The model under review builds one solid part; all positions refer to its coordinate system, in mm. Face numbers are marked on the shaded views. Round coordinates to 2 decimals unless told otherwise and drop trailing zeros. Write each loop counter-clockwise with the first axis right and the second up, starting at its lowest first coordinate (ties: lowest second). Pieces come first, ordered by that corner, then holes.
Item 1: To check wall thickness, follow L1, parallel to Z at x = 17, y = -10; L2, parallel to Z at x = 17.25, y = -72.5; L3, parallel to Y at x = 20.25, z = -44. State the ranges of each line that lie inside material, in increasing order.
Item 2: Draft analysis for pull direction Y (two halves, no side actions). For the marked faces 1, 2, 3 and 4, state which applies: +Y half, -Y half, draft (parallel to the pull), parting line (faces both ways), or undercut.
Item 3: Add section C-C (y = -47.5). Give the boundary of the cut face in (x, z).
Item 4: Add section A-A (x = 12.5). State how many separate pieces and enclosed holes the cut face has, plus the area to 3 significant figures.
Item 5: Add section B-B (y = -10). Give the boundary of the cut face in (x, z), plus the area to 3 significant figures.
Item 6: Clearance check with flat-ended pins moving along their axes: pin 1 Ø5 at (x, y) = (6, -58.5) entering from +Z; pin 2 Ø2 at (y, z) = (-10.5, -35.5) entering from -X; pin 3 Ø13 at (y, z) = (-97.5, -15.95) entering from +X; pin 4 Ø5.5 at (y, z) = (-10, -11) entering from +X. State where each tip first meets the part, or that it passes through.
Item 7: Add section D-D (z = -46). Give the boundary of the cut face in (x, y), plus the area to 4 significant figures.
Autodesk Inventor part; units mm, degrees
ref_plane "YZ Plane" through (0, 0, 0) normal (1, 0, 0) x (0, 1, 0)
ref_plane "XZ Plane" through (0, 0, 0) normal (0, 1, 0) x (-1, 0, 0)
ref_plane "XY Plane" through (0, 0, 0) normal (0, 0, 1) x (1, 0, 0)
sketch "Sketch1" plane through (0, 0, 0) normal (1, 0, 0) x (0, 1, 0)
  line L0 (0, 0) -> (-145, 0)
  line L1 (-145, 0) -> (-145, -70)
  line L2 (-145, -70) -> (0, -70)
  line L3 (0, -70) -> (0, 0)
  dimension "d0" = 145
  dimension "d1" = 70
extrude "Extrusion1" add sketch "Sketch1" along normal blind 20
sketch "Sketch5" plane through (20, 0, 0) normal (1, 0, 0) x (0, 0, -1)
  line L0 (49.9481, -33) -> (-5.5519, -33)
  arc A0 (-6.6519, -32.6703) -> (-5.5519, -33) centre (-5.5519, -31) ccw
  line L1 (-6.6519, -32.6703) -> (-6.6519, -47)
  arc A1 (-9.5519, -49.9) -> (-6.6519, -47) centre (-9.5519, -47) ccw
  line L2 (-9.5519, -49.9) -> (-23.8816, -49.9)
  arc A2 (-23.5519, -51) -> (-23.8816, -49.9) centre (-25.5519, -51) ccw
  line L3 (-23.5519, -51) -> (-23.5519, -106.5)
  arc A3 (-23.5519, -106.5) -> (-18.0519, -112) centre (-18.0519, -106.5) ccw
  line L4 (-18.0519, -112) -> (49.9481, -112)
  arc A4 (49.9481, -112) -> (55.4481, -106.5) centre (49.9481, -106.5) ccw
  line L5 (55.4481, -106.5) -> (55.4481, -38.5)
  arc A5 (55.4481, -38.5) -> (49.9481, -33) centre (49.9481, -38.5) ccw
  circle A6 centre (15.9481, -97.5) radius 1.65
  circle A7 centre (15.9481, -47.5) radius 1.65
  circle A8 centre (50.6979, -96.4808) radius 0.6924
  circle A9 centre (-9.0519, -72.5) radius 5.5
  circle A10 centre (40.9481, -72.5) radius 5.5
  circle A11 centre (15.9481, -72.5) radius 2.5
  circle A12 centre (-9.0519, -97.5) radius 4
  circle A13 centre (40.9481, -47.5) radius 4
  circle A14 centre (28.9481, -89.75) radius 1.5
  circle A15 centre (47.9481, -43.6) radius 1.5
  circle A16 centre (-12.9519, -104.5) radius 1.5
  circle A17 centre (33.1981, -85.5) radius 1.5
  circle A18 centre (-1.8019, -49.6) radius 1.5
  circle A19 centre (-6.9519, -54.75) radius 1.5
  line L6 (43.2888, -99.6225) -> (54.231, -96.5)
  line L7 (54.231, -96.5) -> (50.8902, -107.3775)
  line L8 (50.8902, -107.3775) -> (39.9481, -110.5)
  line L9 (39.9481, -110.5) -> (43.2888, -99.6225)
  line L10 (49.9481, -32.5) -> (-5.5519, -32.5)
  arc A20 (55.9481, -38.5) -> (49.9481, -32.5) centre (49.9481, -38.5) ccw
  line L11 (55.9481, -106.5) -> (55.9481, -38.5)
  arc A21 (49.9481, -112.5) -> (55.9481, -106.5) centre (49.9481, -106.5) ccw
  line L12 (-18.0519, -112.5) -> (49.9481, -112.5)
sketch "Sketch10" plane through (20, 0, 0) normal (1, 0, 0) x (0, 0, -1)
  line L0 (0, 0) -> (0, -145) construction
  line L1 (0, -145) -> (70, -145) construction
  line L2 (70, -145) -> (70, 0) construction
  line L3 (70, 0) -> (0, 0) construction
  line L4 (49.9481, -32.5) -> (-5.5519, -32.5) construction
  line L5 (55.9481, -106.5) -> (55.9481, -38.5) construction
  line L6 (-18.0519, -112.5) -> (49.9481, -112.5) construction
  line L7 (0, 0) -> (0, -145) construction
  line L8 (0, -112.5) -> (0, -145)
  line L9 (0, -145) -> (70, -145)
  line L10 (0, -145) -> (70, -145)
  line L11 (70, -145) -> (70, 0)
  line L12 (70, -145) -> (70, 0)
  line L13 (70, 0) -> (0, 0)
  line L14 (70, 0) -> (0, 0)
  line L15 (0, 0) -> (0, -27.5)
  line L16 (0, -27.5) -> (53.9481, -27.5)
  line L17 (55.9481, -29.5) -> (55.9481, -109.6716)
  line L18 (53.1196, -112.5) -> (0, -112.5)
  arc A0 (55.9481, -29.5) -> (53.9481, -27.5) centre (53.9481, -29.5) ccw
  line L19 (53.1196, -112.5) -> (55.9481, -109.6716) construction
  arc A1 (53.1196, -112.5) -> (55.9481, -109.6716) centre (54.5339, -111.0858) ccw
  dimension "d74" = 85
  dimension "d76" = 2
  dimension "d79" = 45
  dimension "d80" = 4
extrude "Extrusion2" add sketch "Sketch10" along normal blind 2
sketch "Sketch2" plane through (22, 0, 0) normal (1, 0, 0) x (0, 0, -1)
  line L0 (-23.2163, -0.5426) -> (-23.2163, -85.5426) construction
  line L1 (10, -10) -> (60, -10) construction
  line L2 (60, -10) -> (60, -135) construction
  line L3 (60, -135) -> (10, -135) construction
  line L4 (10, -135) -> (10, -10) construction
  line L5 (-23.2163, -85.5426) -> (29.9034, -85.5426)
  arc A0 (29.9034, -85.5426) -> (32.7318, -82.7142) centre (31.3176, -84.1284) ccw
  line L6 (32.7318, -82.7142) -> (32.7318, -2.5426)
  arc A1 (32.7318, -2.5426) -> (30.7318, -0.5426) centre (30.7318, -2.5426) ccw
  line L7 (30.7318, -0.5426) -> (-23.2163, -0.5426)
  line L8 (70, 0) -> (0, 0)
  line L9 (70, -145) -> (70, 0)
  dimension "d4" = 50
  dimension "d5" = 125
  dimension "d81" = 10
  dimension "d82" = 10
hole "M6CBoreToTable" at (22, -10, -10) at (22, -10, -60) at (22, -135, -60) at (22, -135, -10) direction (-1, 0, 0) diameter 6.6 end through all counterbore diameter 11 counterbore depth 6.8
hole "Hole9" at (20, -72.5, -40.9481) direction (-1, 0, 0) diameter 4.917 depth 17.1 tip angle 118
chamfer "Chamfer1" distance 0.5 angle 45 1 edges at (20, -72.5, -38.4896)
sketch "Sketch11" plane through (0, 0, 0) normal (-1, 0, 0) x (0, 0, 1)
  circle A0 centre (-60, -10) radius 3.3 construction
  circle A1 centre (-10, -135) radius 3.3 construction
  line L0 (-60, -10) -> (-10, -10) construction
  line L1 (-10, -10) -> (-10, -135) construction
  line L2 (-10, -135) -> (-60, -135) construction
  line L3 (-60, -135) -> (-60, -10) construction
  circle A2 centre (-35, -10) radius 2
  line L4 (-35, -138) -> (-35, -132) construction
  line L5 (-33, -138) -> (-33, -132)
  line L6 (-37, -132) -> (-37, -138)
  arc A3 (-37, -138) -> (-33, -138) centre (-35, -138) ccw
  arc A4 (-33, -132) -> (-37, -132) centre (-35, -132) ccw
  point P0 (0, 0)
  point P1 (-35, -135)
  dimension "d86" = 4
  dimension "d87" = 3
  dimension "d88" = 4
hole "Hole10" at (0, -10, -35) at (0, -135, -35) at (0, -132, -35) at (0, -138, -35) direction (1, 0, 0) diameter 4 depth 10
extrude "Extrusion3" cut sketch "Sketch11" against normal up to surface (10 mm away) contours A3 L6 A4 L5
sketch "Sketch12" plane through (0, 0, 0) normal (-1, 0, 0) x (0, 0, 1)
  line L0 (-70, -145) -> (-70, 0)
  line L1 (0, -112.5) -> (0, -145)
  line L2 (-70, -20) -> (0, -20)
  line L3 (0, -20) -> (0, -125)
  line L4 (0, -125) -> (-70, -125)
  line L5 (-70, -125) -> (-70, -20)
  line L6 (-70, 0) -> (0, 0)
  line L7 (0, -145) -> (-70, -145)
  dimension "d98" = 20
  dimension "d99" = 20
extrude "Extrusion4" cut sketch "Sketch12" against normal blind 1 contours L0 L2 L3 L1 L4
sketch "Sketch6" plane through (1, 0, 0) normal (-1, 0, 0) x (0, 0, 1)
  point P0 (0, 0)
  point P1 (-15.9481, -47.5)
  point P2 (-15.9481, -97.5)
sketch "Sketch8" plane through (1, 0, 0) normal (-1, 0, 0) x (0, 0, 1)
  circle A0 centre (-15.9481, -72.5) radius 2.5
  point P0 (0, 0)
hole "M6CBoreToMounted" at (1, -72.5, -15.9481) direction (1, 0, 0) diameter 6.6 end through all counterbore diameter 11 counterbore depth 6.8
hole "Hole8" at (1, -47.5, -15.9481) at (1, -97.5, -15.9481) direction (1, 0, 0) diameter 4.5 end through all counterbore diameter 8 counterbore depth 10
equation "\"d86\" = d88"
equation "\"d89\" = d88"
properties part number "FAB-OX0009"
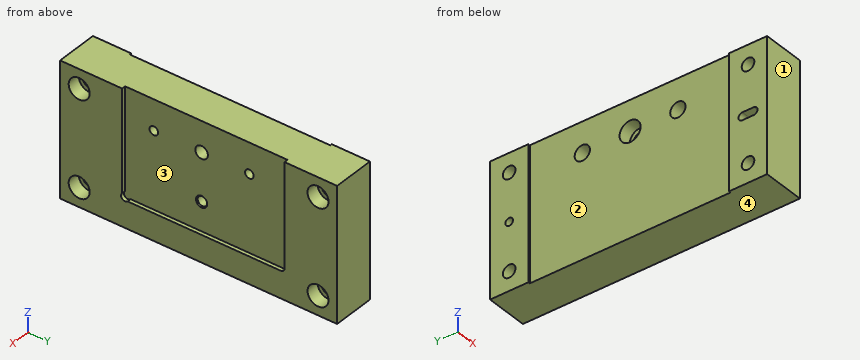
Numbers:
1. L1: z = -70 to -65.5, -54.5 to -15.5, -4.5 to 0
1. L2: z = -70 to -43.41, -38.49 to -19.25, -12.65 to 0
1. L3: y = -145 to -112.5, -27.5 to 0
2. face 1: -Y half
2. face 2: undercut
2. face 3: undercut
2. face 4: draft
3. outline: (1, -70) - (22, -70) - (22, -55.95) - (20, -55.95) - (20, -18.2) - (11, -18.2) - (11, -19.95) - (1, -19.95) - close; (1, -11.95) - (11, -11.95) - (11, -13.7) - (20, -13.7) - (20, 0) - (1, 0) - close
4. separate pieces: 1
4. enclosed holes: 8
4. area: 9,930 mm2
5. outline: (0, -70) - (22, -70) - (22, -65.5) - (15.2, -65.5) - (15.2, -63.3) - (0, -63.3) - close; (0, -56.7) - (15.2, -56.7) - (15.2, -54.5) - (22, -54.5) - (22, -15.5) - (15.2, -15.5) - (15.2, -13.3) - (0, -13.3) - (0, -33) - (10, -33) - (10, -37) - (0, -37) - close; (0, -6.7) - (15.2, -6.7) - (15.2, -4.5) - (22, -4.5) - (22, 0) - (0, 0) - close
5. area: 1,150 mm2
6. pin 1: stops at z = 0
6. pin 2: stops at x = 10
6. pin 3: stops at x = 20
6. pin 4: stops at x = 15.2
7. outline: (0, -145) - (22, -145) - (22, -112.5) - (20, -112.5) - (20, -27.5) - (22, -27.5) - (22, 0) - (0, 0) - (0, -20) - (1, -20) - (1, -125) - (0, -125) - close
7. area: 2,915 mm2
